Check sheet for the drawn part. Datum: minimum x, y, z corner. Units: mm. A direction names the side the tool comes from. Round coordinates to 2 decimals unless told otherwise and drop trailing zeros. Write each loop counter-clockwise with the first axis right and the second up, starting at its lowest first coordinate (ties: lowest second). Pieces come first, ordered by that corner, then holes. Notation, with made-up numbers: (37.25, 37.25) - (79.25, 37.25) arc R22 ccw to (79.25, 52.25) - close; hole circle Ø6 at (37, -8). An arc over 180 degrees is marked (long way). Answer as a JSON object with one key per item and string values. Group by question number.
Item 1: Sectioned sample at A-A on x = 26. Record the boundary of the cut face in (y, z), plus the area to 3 significant figures.
Item 2: Sectioned sample at B-B on z = 85. Record the boundary of the cut face in (x, y).
Item 3: Thickness scan on line 1 (Z direction, x = 26, y = 3); line 2 (Y direction, x = 4.5, z = 115.5); line 3 (Y direction, x = 21, z = 108.5). Record the ranges inside material, lowest first.
Item 4: Set-up check for the marked faces 1 and 2: record each of +Z, -Z, +X, -X, +Y, -Y from which the full face is reachable in a straight line by a thin tool's end or side.
Item 5: Sectioned sample at D-D on y = 4. Record the boundary of the cut face in (x, z).
Item 6: Gauge pin test, flat ends, axial feed: P1, Ø3, axis at y = 30, z = 152, coming from the +X side; P2, Ø5, axis at x = 5.5, z = 86, coming from the +Y side; P3, Ø1.8, axis at x = 17, y = 4, coming from the +Z side; P4, Ø9, axis at x = 26, z = 85, coming from the +Y side (3 decimals). Record the tip position at first contact, or that the pin passes through.
Item 7: Sectioned sample at C-C on y = 35. Record the boundary of the cut face in (x, z), plus the area to 3 significant figures.
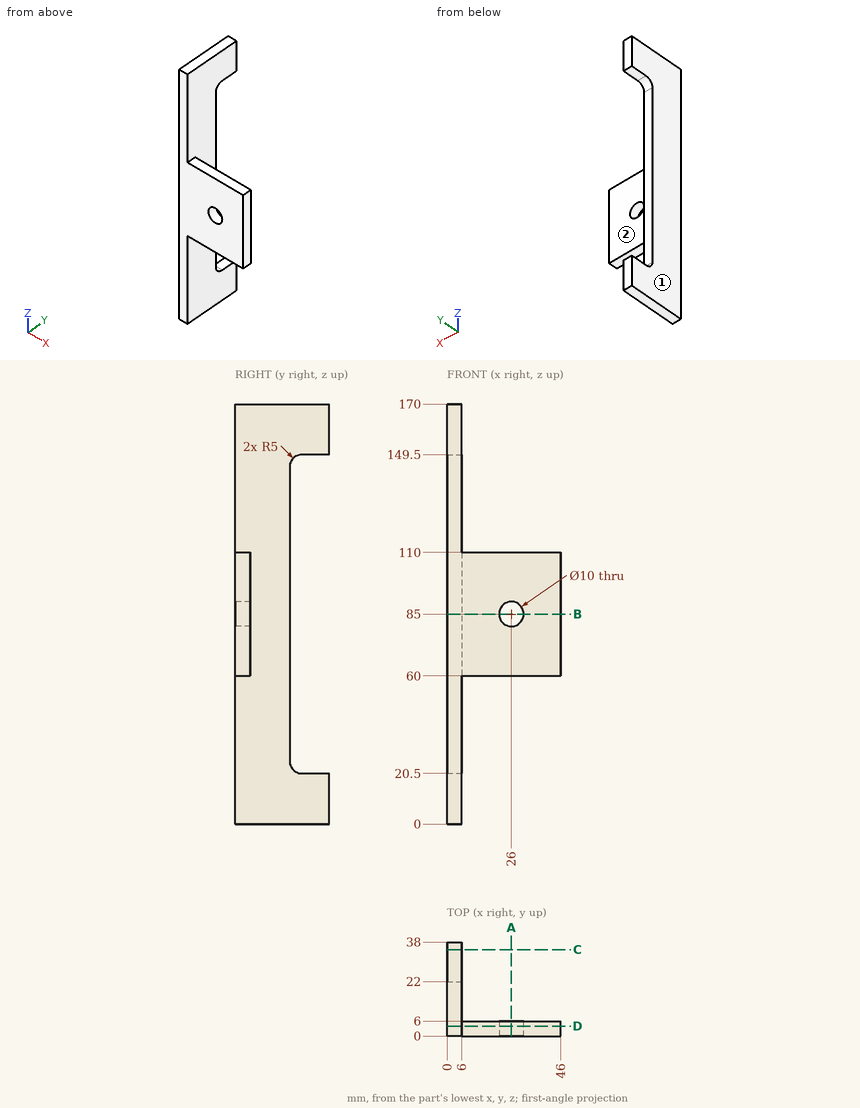
Completed:
{
 "1": {"outline": "(0, 60) - (6, 60) - (6, 80) - (0, 80) - close; (0, 90) - (6, 90) - (6, 110) - (0, 110) - close", "area": "240 mm²"},
 "2": {"outline": "(0, 0) - (21, 0) - (21, 6) - (6, 6) - (6, 22) - (0, 22) - close; (31, 0) - (46, 0) - (46, 6) - (31, 6) - close"},
 "3": {"line 1": "60 to 80, 90 to 110", "line 2": "0 to 22", "line 3": "0 to 6"},
 "4": {"face 1": "+Z, -Z, -X, +Y, -Y", "face 2": "+Z, -Z, +X, +Y"},
 "5": {"outline": "(0, 0) - (6, 0) - (6, 60) - (46, 60) - (46, 110) - (6, 110) - (6, 170) - (0, 170) - close; hole circle Ø10 at (26, 85)"},
 "6": {"P1": "x = 6", "P2": "y = 22", "P3": "z = 110", "P4": "through"},
 "7": {"outline": "(0, 0) - (6, 0) - (6, 20.5) - (0, 20.5) - close; (0, 149.5) - (6, 149.5) - (6, 170) - (0, 170) - close", "area": "246 mm²"}
}
